Verification items for the finished model (mm, model axes). A direction names the side the tool comes from. Give positions to 0.01 mm unless a question says otherwise; leave off trailing zeros. Write each loop counter-clockwise with the first axis right and the second up, starting at its lowest first coordinate (ties: lowest second). Pieces come first, ordered by that corner, then holes. Notation, with made-up numbers: (52, 49.5) -> (62, 49.5) arc R16 ccw to (62, 60.5) -> close; hole circle Ø4 at (15.5, 84). An arc over 180 degrees is marked (long way). Answer as CSV lines item,"result".
```python
from build123d import *

# Parameters (mm, degrees)
CUT_EXTRUDE_1_REACH      = 68.168
SKETCH_5_R               = 1.75
PATTERN_CIRCULAR_2_COUNT = 8
PATTERN_CIRCULAR_3_COUNT = 2
PATTERN_CIRCULAR_3_ANGLE = 30
SKETCH_9_R               = 18
SKETCH_9_R_2             = 10
EXTRUDE_1_DEPTH          = 5.5
PATTERN_CIRCULAR_4_COUNT = 3
SKETCH_12_R              = 12.742570665
SKETCH_12_R_2            = 9.958698881
CUT_EXTRUDE_2_DEPTH      = 0.5
CUT_EXTRUDE_START        = -0.5
SKETCH_13_R              = 11.804980978
SKETCH_13_R_2            = 10
CUT_EXTRUDE_3_DEPTH      = 0.5
PATTERN_CIRCULAR_5_COUNT = 4
PATTERN_CIRCULAR_6_COUNT = 4


with BuildPart() as part:
    # 草图1 → 旋转1 (revolve)
    with BuildSketch(Plane.XY, mode=Mode.PRIVATE) as revolve_1_sk:
        Polygon((0, 7), (0, 10), (12, 10), (12, 37), (21, 37), (21, 35), (32.5, 35), (32.5, 27), (37, 24.401923789), (37, 27), (45, 27), (45, 18), (52.5, 18), (52.5, 7), align=None)
    revolve(revolve_1_sk.sketch.rotate(Axis((-65.200779727, 0, 0), (1, 0, 0)), 90), axis=Axis((-65.200779727, 0, 0), (1, 0, 0)))

    # 草图5 → 切除-拉伸1 (cut, up to next)
    with BuildSketch(Plane.ZY.offset(-12), mode=Mode.PRIVATE) as cut_extrude_1_sk1:
        with Locations((0, 32)):
            Circle(SKETCH_5_R)
    cut_extrude_1_tool1 = extrude(cut_extrude_1_sk1.sketch, amount=-CUT_EXTRUDE_1_REACH, mode=Mode.PRIVATE) & part.part
    cut_extrude_1 = cut_extrude_1_tool1.solids().sort_by_distance((12, 32, 0))[0]
    add(cut_extrude_1, mode=Mode.SUBTRACT)

    # 阵列(圆周)2: 切除-拉伸1 ×8 about axis
    pattern_circular_2_axis = Axis((0, 0, 0), (1, 0, 0))
    for i in range(1, PATTERN_CIRCULAR_2_COUNT):
        add(cut_extrude_1.rotate(pattern_circular_2_axis, i * 360 / PATTERN_CIRCULAR_2_COUNT), mode=Mode.SUBTRACT)

    # 草图7 → M3 螺纹孔2 (revolve, cut)
    with BuildSketch(Plane(origin=(45, 22, 0), x_dir=(0, 0, -1), z_dir=(0, 1, 0))):
        Polygon((0, 0), (0, 12.251075774), (1.25, 11.5), (1.25, 0), align=None)
    hole_wizard_m3_2 = revolve(axis=Axis((51.35, 22, 0), (-1, 0, 0)), mode=Mode.SUBTRACT)

    # 阵列(圆周)3: M3 螺纹孔2 ×2 about axis
    pattern_circular_3_axis = Axis((52.5, 0, 0), (-1, 0, 0))
    for i in range(1, PATTERN_CIRCULAR_3_COUNT):
        add(hole_wizard_m3_2.rotate(pattern_circular_3_axis, i * PATTERN_CIRCULAR_3_ANGLE / (PATTERN_CIRCULAR_3_COUNT - 1)), mode=Mode.SUBTRACT)

    # 草图9 → 凸台-拉伸1 (add)
    with BuildSketch(Plane.ZY.offset(-12)):
        Circle(SKETCH_9_R)
        Circle(SKETCH_9_R_2, mode=Mode.SUBTRACT)
    extrude(amount=EXTRUDE_1_DEPTH)

    # 草图10 → M3 螺纹孔3 (revolve, cut)
    with BuildSketch(Plane(origin=(2.5, 10, 0), x_dir=(0, 0, 1), z_dir=(1, 0, 0))):
        Polygon((0, 0), (0, 7.251075774), (1.25, 6.5), (1.25, 0), align=None)
    hole_wizard_m3_3 = revolve(axis=Axis((2.5, 16.35, 0), (0, -1, 0)), mode=Mode.SUBTRACT)

    # 阵列(圆周)4: M3 螺纹孔3 ×3 about axis
    pattern_circular_4_axis = Axis((52.5, 0, 0), (-1, 0, 0))
    for i in range(1, PATTERN_CIRCULAR_4_COUNT):
        add(hole_wizard_m3_3.rotate(pattern_circular_4_axis, i * 360 / PATTERN_CIRCULAR_4_COUNT), mode=Mode.SUBTRACT)

    # 草图12 → 切除-拉伸2 (cut)
    with BuildSketch(Plane(origin=(52.5, 0, 0), x_dir=(0, 0, -1), z_dir=(1, 0, 0))):
        Circle(SKETCH_12_R)
        Circle(SKETCH_12_R_2, mode=Mode.SUBTRACT)
    extrude(amount=-CUT_EXTRUDE_2_DEPTH, mode=Mode.SUBTRACT)

    # 草图13 → 切除-拉伸3 (cut)
    with BuildSketch(Plane.ZY.offset(-6.5).offset(CUT_EXTRUDE_START)):
        Circle(SKETCH_13_R)
        Circle(SKETCH_13_R_2, mode=Mode.SUBTRACT)
    extrude(amount=CUT_EXTRUDE_3_DEPTH, mode=Mode.SUBTRACT)

    # 阵列(圆周)5: M3 螺纹孔2 ×4 about axis
    pattern_circular_5_axis = Axis((0, 0, 0), (1, 0, 0))
    for i in range(1, PATTERN_CIRCULAR_5_COUNT):
        add(hole_wizard_m3_2.rotate(pattern_circular_5_axis, i * 360 / PATTERN_CIRCULAR_5_COUNT), mode=Mode.SUBTRACT)

    # 阵列(圆周)5 copy 1 sketch → 阵列(圆周)5 copy 1 (revolve, cut)
    with BuildSketch(Plane(origin=(45, 11, 19.052558883), x_dir=(0, 0.866025403784438, -0.5000000000000011), z_dir=(0, 0.5000000000000011, 0.866025403784438))):
        Polygon((0, 0), (0, 12.251075774), (1.25, 11.5), (1.25, 0), align=None)
    revolve(axis=Axis((51.35, 11, 19.052558883), (-1, 0, 0)), mode=Mode.SUBTRACT)

    # 阵列(圆周)5 copy 2 sketch → 阵列(圆周)5 copy 2 (revolve, cut)
    with BuildSketch(Plane(origin=(45, -19.052558883, 11), x_dir=(0, 0.5000000000000012, 0.8660254037844379), z_dir=(0, -0.8660254037844379, 0.5000000000000012))):
        Polygon((0, 0), (0, 12.251075774), (1.25, 11.5), (1.25, 0), align=None)
    revolve(axis=Axis((51.35, -19.052558883, 11), (-1, 0, 0)), mode=Mode.SUBTRACT)

    # 阵列(圆周)5 copy 3 sketch → 阵列(圆周)5 copy 3 (revolve, cut)
    with BuildSketch(Plane(origin=(45, -11, -19.052558883), x_dir=(0, -0.8660254037844379, 0.5000000000000012), z_dir=(0, -0.5000000000000012, -0.8660254037844379))):
        Polygon((0, 0), (0, 12.251075774), (1.25, 11.5), (1.25, 0), align=None)
    revolve(axis=Axis((51.35, -11, -19.052558883), (-1, 0, 0)), mode=Mode.SUBTRACT)

    # 草图14 → 打孔尺寸(%根据)内六角圆柱头螺钉的类型1 (revolve, cut)
    with BuildSketch(Plane(origin=(45, 11, -19.052558883), x_dir=(0, 0, -1), z_dir=(0, 1, 0))):
        Polygon((0, 0), (0, 16.521463052), (1.7, 15.5), (1.7, 3.4), (3, 3.4), (3, 0), align=None)
    hole_wizard_1 = revolve(axis=Axis((51.35, 11, -19.052558883), (-1, 0, 0)), mode=Mode.SUBTRACT)

    # 阵列(圆周)6: 打孔尺寸(%根据)内六角圆柱头螺钉的类型1 ×4 about axis
    pattern_circular_6_axis = Axis((0, 0, 0), (1, 0, 0))
    for i in range(1, PATTERN_CIRCULAR_6_COUNT):
        add(hole_wizard_1.rotate(pattern_circular_6_axis, i * 360 / PATTERN_CIRCULAR_6_COUNT), mode=Mode.SUBTRACT)


solid = part.part
```
1) Depth check by flat-ended pin: pin 1 (5.5 mm diameter, centred on y = -19.05, z = -11, fed in from -X); pin 2 (3 mm diameter, centred on y = -11, z = 5.5, fed in from +X); pin 3 (5.5 mm diameter, centred on y = 22.63, z = 22.63, fed in from +X); pin 4 (12 mm diameter, centred on x = 32.5, y = -13, fed in from +Z). Enter the tip coordinate at first touch or a pass-through.
Reported:
pin 1,"x = 12"
pin 2,"x = 52.5"
pin 3,"x = 32.5"
pin 4,"z = 34.29"
2) Section check B-B (x = 2.5). Record the boundary of the cut face in (y, z).
Reported:
outline,"(-6.04, -7.97) -> (-4.53, -5.34) arc R7 cw to (-4.53, 5.34) -> (-6.04, 7.97) arc R10 ccw to start; (-3.88, -9.22) arc R10 ccw to (9.92, -1.25) -> (6.89, -1.25) arc R7 cw to (-2.36, -6.59) -> close; (-3.88, 9.22) -> (-2.36, 6.59) arc R7 cw to (6.89, 1.25) -> (9.92, 1.25) arc R10 ccw to start"
3) Section check A-A (y = -32). Record the boundary of the cut face in (x, z), and give its area (3 significant figures).
Reported:
outline,"(12, -18.57) -> (21, -18.57) -> (21, -14.18) -> (32.5, -14.18) -> (32.5, -1.75) -> (12, -1.75) -> close; (12, 1.75) -> (32.5, 1.75) -> (32.5, 14.18) -> (21, 14.18) -> (21, 18.57) -> (12, 18.57) -> close"
area,"589 mm²"
4) Scan lines: line 1 along X through (y, z) = (20.5, -19); line 2 along Y through (x, z) = (34, 5); line 3 along Z through (x, y) = (38, 1). Record each from-to range of solid material in increasing order.
Reported:
line 1,"12 to 32.5"
line 2,"-25.65 to -4.9, 4.9 to 25.65"
line 3,"-26.98 to -22.75, -21.25 to -6.93, 6.93 to 21.25, 22.75 to 26.98"
5) Section check C-C (x = 44). State how many separate pieces and enclosed holes the cut face has, and give its area (3 significant figures).
Reported:
separate pieces,"1"
enclosed holes,"13"
area,"1,980 mm²"
6) Draft check along Z on faces 1 (the flat face through (32.5, 8, -26)), 2 (the cylindrical face through (39.33, -23.22, -0.27)), 3 (the cylindrical face through (48.802, -12.165, -13.267)). Enter one of: +Z half, -Z half, draft (parallel to the pull), parting line (faces both ways), or undercut.
Reported:
face 1,"draft"
face 2,"undercut"
face 3,"parting line"
7) Tool access check on faces 4 (the cylindrical face through (39.33, -11.845, -18.131)), 5 (the cylindrical face through (6.754, -11.524, -2.559)), 6 (the cylindrical face through (1.26, 8.46, -0.16)). Record the directions out of +Z, -Z, +X, -X, +Y, -Y that give a thin tool (end or side, any length) a straight path to the whole face; none if there is none.
Reported:
face 4,"+X"
face 5,"-X"
face 6,"+Y"
